Here's the drawing with two shaded views (mm, measured from the low corner). I have some questions. A direction names the side the tool comes from. Coordinates: 2 decimals unless noted, no trailing zeros. Loops run counter-clockwise (first coordinate to the right, second up) from the corner with the lowest first, then second, coordinate; pieces in that order, holes last. Notation, with made-up numbers: (63.25, 47) -> (109.25, 47) arc R27 ccw to (109.25, 77) -> close; hole circle Ø7 at (29, -35). An arc over 180 degrees is marked (long way). Answer as a JSON object with one key per item and string values. Group by question number.
Q1. I want a section at A-A on y = 5.5. Write out the boundary of the cut face in (x, z), then the cut area to 3 significant figures.
Q2. I'm going to push flat-ended pins straight in: pin 1 (10 mm diameter, centred on x = 5.5, y = 5, fed in from +Z); pin 2 (1.5 mm diameter, centred on x = 13.75, z = 22.75, fed in from -Y); pin 3 (1.2 mm diameter, centred on x = 14, z = 22, fed in from -Y). Where does each tip first touch, or does it pass through?
Q3. On a 3-axis mill with a long thin cutter (end or side, diameter ignored), from which of +Z, -Z, +X, -X, +Y, -Y can I reach the whole of each face in a straight line? I mean the marked faces 1 and 2. Say none if no direction works.
Q4. I want a section at B-B on x = 13.75. Write out the boundary of the cut face in (y, z), then the cut area to 3 significant figures.
Q5. I want a section at D-D on y = 26. Write out the boundary of the cut face in (x, z).
Q6. I need wall thicknesses on line 1 (X direction, y = 5.9, z = 13.75); line 2 (X direction, y = 27, z = 13.75); line 3 (Y direction, x = 6, z = 21). Which ranges of each line are inside material? Lowest first, please.
Q7. I want a section at C-C on z = 13.75. Write out the boundary of the cut face in (x, y), then the cut area to 3 significant figures.
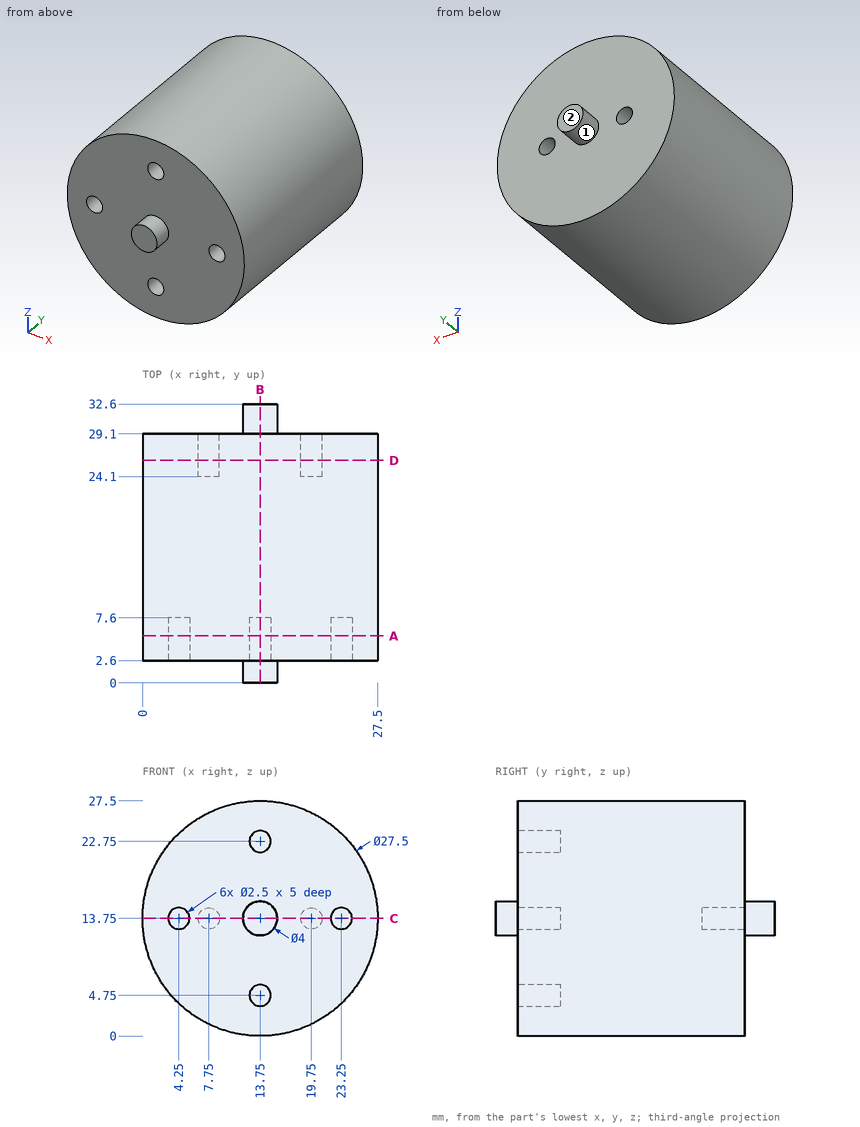
Result set:
{
 "1": {"outline": "circle Ø27.5 at (13.75, 13.75); hole circle Ø2.5 at (4.25, 13.75); hole circle Ø2.5 at (13.75, 4.75); hole circle Ø2.5 at (13.75, 22.75); hole circle Ø2.5 at (23.25, 13.75)", "area": "574 mm²"},
 "2": {"pin 1": "stops at z = 27.11", "pin 2": "stops at y = 7.6", "pin 3": "stops at y = 2.6"},
 "3": {"face 1": "+Y", "face 2": "+Z, -Z, +X, -X, +Y"},
 "4": {"outline": "(0, 11.75) -> (2.6, 11.75) -> (2.6, 6) -> (7.6, 6) -> (7.6, 3.5) -> (2.6, 3.5) -> (2.6, 0) -> (29.1, 0) -> (29.1, 11.75) -> (32.6, 11.75) -> (32.6, 15.75) -> (29.1, 15.75) -> (29.1, 27.5) -> (2.6, 27.5) -> (2.6, 24) -> (7.6, 24) -> (7.6, 21.5) -> (2.6, 21.5) -> (2.6, 15.75) -> (0, 15.75) -> close", "area": "728 mm²"},
 "5": {"outline": "circle Ø27.5 at (13.75, 13.75); hole circle Ø2.5 at (7.75, 13.75); hole circle Ø2.5 at (19.75, 13.75)"},
 "6": {"line 1": "x = 0 to 3, 5.5 to 22, 24.5 to 27.5", "line 2": "x = 0 to 6.5, 9 to 18.5, 21 to 27.5", "line 3": "y = 2.6 to 29.1"},
 "7": {"outline": "(0, 2.6) -> (3, 2.6) -> (3, 7.6) -> (5.5, 7.6) -> (5.5, 2.6) -> (11.75, 2.6) -> (11.75, 0) -> (15.75, 0) -> (15.75, 2.6) -> (22, 2.6) -> (22, 7.6) -> (24.5, 7.6) -> (24.5, 2.6) -> (27.5, 2.6) -> (27.5, 29.1) -> (21, 29.1) -> (21, 24.1) -> (18.5, 24.1) -> (18.5, 29.1) -> (15.75, 29.1) -> (15.75, 32.6) -> (11.75, 32.6) -> (11.75, 29.1) -> (9, 29.1) -> (9, 24.1) -> (6.5, 24.1) -> (6.5, 29.1) -> (0, 29.1) -> close", "area": "703 mm²"}
}
